```python
from build123d import *

# Parameters (mm, degrees)
SKETCH1_W           = 254
SKETCH1_H           = 101.6
SKETCH1_R           = 25.4
BOSS_EXTRUDE1_DEPTH = 3.175
SKETCH2_R           = 3.175
CUT_EXTRUDE1_DEPTH  = 7.35
CIRPATTERN1_COUNT   = 5


with BuildPart() as part:
    # Sketch1 → Boss-Extrude1 (new body, symmetric)
    with BuildSketch(Plane(origin=(0, 0, 0), x_dir=(0, 0, -1), z_dir=(1, 0, 0))):
        Rectangle(SKETCH1_W, SKETCH1_H)
        with Locations((-63.5, 0)):
            Circle(SKETCH1_R, mode=Mode.SUBTRACT)
    extrude(amount=BOSS_EXTRUDE1_DEPTH, both=True)

    # Sketch2 → Cut-Extrude1 (cut, through all)
    with BuildSketch(Plane(origin=(3.175, 0, 0), x_dir=(0, 0, -1), z_dir=(1, 0, 0))):
        with Locations((-63.5, 38.1)):
            Circle(SKETCH2_R)
    cut_extrude1 = extrude(amount=-CUT_EXTRUDE1_DEPTH, mode=Mode.SUBTRACT)

    # CirPattern1: Cut-Extrude1 ×5 about axis
    cirpattern1_axis = Axis((0, 0, 63.5), (1, 0, 0))
    for i in range(1, CIRPATTERN1_COUNT):
        add(cut_extrude1.rotate(cirpattern1_axis, i * 360 / CIRPATTERN1_COUNT), mode=Mode.SUBTRACT)


solid = part.part
```
Source: CAD feature listing. Evaluate the final solid. Frame: model axes, mm. Round coordinates to 2 decimals unless told otherwise and drop trailing zeros. Loops run counter-clockwise (first coordinate to the right, second up) from the corner with the lowest first, then second, coordinate; pieces in that order, holes last. Notation, with made-up numbers: M -32,-36 L -1,-36 A12 cw -1,-25 Z; hole C 29,-23.5 d1. An arc over 180 degrees is marked long. Use a Markdown table: item, result. Add a question column.
1. Section query A-A on y = 0. Return the cut outline in (x, z) (3 decimals).
2. Section query D-D on x = 1.75. Return the cut outline in (y, z) (3 decimals).
3. Contact query for a flat-ended pin moving along its axis: P1, Ø7.5, axis at y = -30.82, z = 85.89, coming from the +X side (3 decimals). Output: stop coordinate, or through.
4. Mould query, pull axis Z, two halves, no side actions, for faces 1 (the cylindrical face through (0, -15, 84)), 2 (the flat face through (0, -1, 127)), 3 (the flat face through (0, -50.8, 2)). Classes: pulls with the +Z half, pulls with the -Z half, needs draft (parallel to the pull), parting line crosses it, or undercut.
5. Section query C-C on y = 38.1. Return the cut outline in (x, z) (3 decimals), then the cut area to 3 significant figures.
6. Section query B-B on z = 63.5. Return the cut outline in (x, y) (3 decimals).
7. Line query: line 1 (Y direction, x = 1.5, z = 63.5) (3 decimals); line 2 (Y direction, x = -0.5, z = 85.5); line 3 (Y direction, x = -2.75, z = 25). Output: solid intervals per line, ascending.
Reported:
| question | item | result |
|---|---|---|
| 1 | outline | M -3.175,-127 L 3.175,-127 L 3.175,38.1 L -3.175,38.1 Z; M -3.175,88.9 L 3.175,88.9 L 3.175,127 L -3.175,127 Z |
| 2 | outline | M -50.8,-127 L 50.8,-127 L 50.8,127 L -50.8,127 Z; hole C -30.824,41.105 d6.35; hole C -30.824,85.895 d6.35; hole C 0,63.5 d50.8; hole C 11.774,27.265 d6.35; hole C 11.774,99.735 d6.35; hole C 38.1,63.5 d6.35 |
| 3 | P1 | stops at x = 3.175 |
| 4 | face 1 | undercut |
| 4 | face 2 | pulls with the +Z half |
| 4 | face 3 | needs draft |
| 5 | outline | M -3.175,-127 L 3.175,-127 L 3.175,60.325 L -3.175,60.325 Z; M -3.175,66.675 L 3.175,66.675 L 3.175,127 L -3.175,127 Z |
| 5 | area | 1,570 mm² |
| 6 | outline | M -3.175,-50.8 L 3.175,-50.8 L 3.175,-25.4 L -3.175,-25.4 Z; M -3.175,25.4 L 3.175,25.4 L 3.175,34.925 L -3.175,34.925 Z; M -3.175,41.275 L 3.175,41.275 L 3.175,50.8 L -3.175,50.8 Z |
| 7 | line 1 | y = -50.8 to -25.4, 25.4 to 34.925, 41.275 to 50.8 |
| 7 | line 2 | y = -50.8 to -33.97, -27.67 to -12.69, 12.69 to 50.8 |
| 7 | line 3 | y = -50.8 to 9.55, 14 to 50.8 |
